The model under review builds one solid part; all positions refer to its coordinate system, in mm. Give positions to 0.01 mm unless a question says otherwise; leave off trailing zeros. Answer as a JSON object with one key per item and string values.
from build123d import *

# Parameters (mm, degrees)
SKETCH18_R         = 2.1844
CUT_EXTRUDE1_DEPTH = 314.841780485


with BuildPart() as part:
    # Loft1: read off the stored shape, not the designer's step
    # Loft1: loft between two sections, ruled curve by curve
    loft1_from = [
        Edge.make_bspline([(56.833832956, 0, -228.6), (56.833832956, -24.296302856, -228.6), (37.93302454, -48.592605712, -228.6), (-37.670209127, -48.592605712, -228.6), (-56.571017544, -24.296302856, -228.6), (-56.571017544, 0, -228.6)], [0, 0, 0, 0, 0.5, 0.5, 1, 1, 1, 1], 3, [1, 0.666666667, 0.5, 0.5, 0.666666667, 1]),
        Edge.make_bspline([(-52.761017544, 0, -228.6), (-52.761017544, -4.747279447, -228.6), (-51.402770393, -11.806188932, -228.6), (-45.595697561, -23.613386766, -228.6), (-39.795169121, -29.862955228, -228.6), (-30.718583767, -36.674634262, -228.6), (-20.272155915, -42.261246959, -228.6), (-8.609583282, -44.495586175, -228.6), (5.258963144, -45.021190556, -228.6), (17.65948625, -43.279675379, -228.6), (30.464702909, -37.058928058, -228.6), (38.535712181, -31.060250812, -228.6), (44.862969288, -24.583491802, -228.6), (51.190783343, -13.941223772, -228.6), (53.023832956, -5.077291503, -228.6), (53.023832956, 0, -228.6)], [0, 0, 0, 0, 0.092670327, 0.138032037, 0.255929417, 0.255929417, 0.359592664, 0.484831486, 0.484831486, 0.630530284, 0.725178151, 0.760432961, 0.82657985, 0.900919869, 1, 1, 1, 1], 3),
        Edge.make_bspline([(53.023832956, 0, -228.6), (53.658832956, 0, -228.6), (54.293832956, 0, -228.6), (55.563832956, 0, -228.6), (56.198832956, 0, -228.6), (56.833832956, 0, -228.6)], [0, 0, 0, 0, 0.5, 0.5, 1, 1, 1, 1], 3),
        Edge.make_line((-52.761017544, 0, -228.6), (-56.571017544, 0, -228.6)),
    ]
    loft1_to = [
        Edge.make_bspline([(56.854039108, 0.001519688, -304.8), (56.855077905, -28.463722616, -304.8), (33.368424055, -48.592160594, -304.8), (-33.063422969, -48.593050818, -304.8), (-56.550811364, -28.465242318, -304.8), (-56.550811364, 0, -304.8)], [0, 0, 0, 0, 0.5, 0.5, 1, 1, 1, 1], 3, [1, 0.647597082, 0.521143499, 0.521143499, 0.647597082, 1]),
        Edge.make_bspline([(-52.740811364, 0, -304.8), (-52.740749216, -4.747279446, -304.8), (-51.382409655, -11.80617115, -304.8), (-45.575182253, -23.613292961, -304.8), (-39.774571999, -29.862785486, -304.8), (-30.697897472, -36.674345695, -304.8), (-20.251396485, -42.260821635, -304.8), (-8.588794603, -44.495008174, -304.8), (5.279758702, -45.020430998, -304.8), (17.680259009, -43.278753482, -304.8), (30.485394229, -37.057838525, -304.8), (38.556324971, -31.059055621, -304.8), (44.883497288, -24.582213779, -304.8), (51.211172022, -13.939862911, -304.8), (53.044105595, -5.075906646, -304.8), (53.044039127, 0.001384857, -304.8)], [0, 0, 0, 0, 0.092670327, 0.138032037, 0.255929417, 0.255929417, 0.359592664, 0.484831486, 0.484831486, 0.630530284, 0.725178151, 0.760432961, 0.82657985, 0.900919869, 1, 1, 1, 1], 3),
        Edge.make_bspline([(53.044039127, 0.001384857, -304.8), (53.679039124, 0.001407329, -304.8), (54.31403912, 0.001429801, -304.8), (55.584039114, 0.001474744, -304.8), (56.219039111, 0.001497216, -304.8), (56.854039108, 0.001519688, -304.8)], [0, 0, 0, 0, 0.5, 0.5, 1, 1, 1, 1], 3),
        Edge.make_line((-52.740811364, 0, -304.8), (-56.550811364, 0, -304.8)),
    ]
    loft1 = Solid(Shell([*[Face.make_surface_from_curves(loft1_from[k], loft1_to[k]) for k in range(4)], Face(Wire(loft1_from)), Face(Wire(loft1_to))]))
    add(loft1)

    # Sketch18 → Cut-Extrude1 (cut, through all)
    with BuildSketch(Plane(origin=(0, 0, 0), x_dir=(1, 0, 0), z_dir=(0, 1, 0))):
        with Locations(Location((25.383246846, 236.22, 0), (0, 0, 270))):
            Circle(SKETCH18_R)
        with Locations(Location((-25.416737266, 236.260177413, 0), (0, 0, 270))):
            Circle(SKETCH18_R)
    extrude(amount=-CUT_EXTRUDE1_DEPTH, mode=Mode.SUBTRACT)


solid = part.part
Q1. The part is to be moulded in two halves that separate along Z. For faces 1 (the face through (0, -46, -304.8)), 2 (the face through (27.23, -41.29, -235.05)), 3 (the face through (0, -46, -228.6)), say which applies: +Z half, -Z half, draft (parallel to the pull), parting line (faces both ways), or undercut.
Results:
{"face 1": "-Z half", "face 2": "undercut", "face 3": "+Z half"}
Q2. Clearance check with flat-ended pins moving along their axes: pin 1 Ø6 at (x, z) = (7.5, -275) entering from -Y; pin 2 Ø2.5 at (x, z) = (-25.42, -236.26) entering from -Y; pin 3 Ø3 at (y, z) = (-13.5, -254.5) entering from -X; pin 4 Ø3 at (y, z) = (-24, -247.5) entering from +X. State where each tip first meets the part, or that it passes through.
Results:
{"pin 1": "stops at y = -48.45", "pin 2": "passes through", "pin 3": "stops at x = -54.8", "pin 4": "stops at x = 50.38"}
Q3. To check wall thickness, follow probe 1 along X at (y, z) = (-25, -245); probe 2 along X at (y, z) = (-19, -243); probe 3 along Y at (x, z) = (6, -254.5). State the ranges of each line that lie inside material, in increasing order. Write a range as [from, to].
Results:
{"probe 1": "x = [-48.47, -43.73], [44, 48.74]", "probe 2": "x = [-52.05, -47.75], [48.02, 52.32]", "probe 3": "y = [-48.33, -44.51]"}
Q4. Consider section A-A, the plane z = -236.22. State how many separate pieces and enclosed holes the cut face has, plus the area to 3 significant figures.
Results:
{"separate pieces": "3", "enclosed holes": "0", "area": "571 mm^2"}
